from build123d import *

# Parameters (mm, degrees)
CROQUIS1_R              = 6
CROQUIS1_R_2            = 13
SALIENTE_EXTRUIR1_DEPTH = 9.525
CROQUIS2_R              = 13
CROQUIS2_R_2            = 7.5
SALIENTE_EXTRUIR2_DEPTH = 1.525


with BuildPart() as part:
    # Croquis1 → Saliente-Extruir1 (new body)
    with BuildSketch(Plane.XY):
        with BuildLine():
            Line((0, 19), (120, 19))
            ThreePointArc((120, 19), (139, 0), (120, -19))
            Line((120, -19), (0, -19))
            ThreePointArc((0, -19), (-19, 0), (0, 19))
        make_face()
        with Locations(Location((0, 0, 0), (0, 0, 180))):
            Circle(CROQUIS1_R, mode=Mode.SUBTRACT)
        with Locations(Location((120, 0, 0), (0, 0, 180))):
            Circle(CROQUIS1_R_2, mode=Mode.SUBTRACT)
    extrude(amount=SALIENTE_EXTRUIR1_DEPTH)

    # Croquis2 → Saliente-Extruir2 (add)
    with BuildSketch(Plane(origin=(0, 0, 0), x_dir=(-1, 0, 0), z_dir=(0, 0, -1))):
        with Locations((-120, 0)):
            Circle(CROQUIS2_R)
        with Locations((-120, 0)):
            Circle(CROQUIS2_R_2, mode=Mode.SUBTRACT)
    extrude(amount=-SALIENTE_EXTRUIR2_DEPTH)


solid = part.part
The listing builds one solid part. Answer for the finished solid, in the listing's coordinates (mm). A direction names the side the tool comes from. Round coordinates to 2 decimals unless told otherwise and drop trailing zeros. Order: outer loops, then holes, each group sorted by start corner. A loop starts at its lowest first (then second) coordinate and runs counter-clockwise, first axis right, second up. Notation, with made-up numbers: M 15.25,-21 L 44.25,-21 A29 ccw 44.25,4 Z; hole C -20.75,51 d10. An arc over 180 degrees is marked long. Answer in a Markdown table with one row per item. Add a question column.
1) Consider line 1 along Y through (x, z) = (120, 3.5); line 2 along Y through (x, z) = (0, 6.25); line 3 along X through (y, z) = (-5, 1.25). Determine where each line is inside the solid, lowest interval first. Write a range as from..to.
2) The part is cut by section B-B on z = 4.25. Determine the outline of the cut face in (x, y), plus the area to 3 significant figures.
3) Flat-ended cylindrical pins translate along their axes: pin 1 Ø4 at (y, z) = (14.5, 2.5) entering from +X; pin 2 Ø12 at (x, y) = (120, 0) entering from -Z; pin 3 Ø5 at (y, z) = (-3.5, 6.5) entering from +X; pin 4 Ø8 at (x, y) = (114, 6.5) entering from +Z (3 decimals). Find the tip coordinate at first contact, or state that the pin passes through.
4) The part is cut by section D-D on y = -16. Determine the outline of the cut face in (x, z) (3 decimals).
5) The part is cut by section C-C on x = -4. Determine the outline of the cut face in (y, z) (3 decimals), plus the area to 3 significant figures.
6) The part is cut by section A-A on y = 0. Determine the outline of the cut face in (x, z) (3 decimals), plus the area to 3 significant figures.
7) Which of the six approach directions +Z, -Z, +X, -X, +Y, -Y give full straight-line access (tool end or side, diameter ignored) to faces 1 (the face through (114, -6, 1.525)), 2 (the face through (-19, 0, 5))?
8) Determine the mould class of faces 3 (the face through (59, 19, 5)), 4 (the face through (61, 0, 0)), 5 (the face through (61, 0, 9.525)) for opening direction Z: pulls with the +Z half, pulls with the -Z half, needs draft (parallel to the pull), parting line crosses it, or undercut.
Findings below:
| question | item | result |
|---|---|---|
| 1 | line 1 | y = -19..-13, 13..19 |
| 1 | line 2 | y = -19..-6, 6..19 |
| 1 | line 3 | x = -18.33..-3.32, 3.32..114.41, 125.59..138.33 |
| 2 | outline | M 0,-19 L 120,-19 A19 ccw 120,19 L 0,19 A19 ccw Z; hole C 0,0 d12; hole C 120,0 d26 |
| 2 | area | 5,050 mm² |
| 3 | pin 1 | stops at x = 134.31 |
| 3 | pin 2 | passes through |
| 3 | pin 3 | stops at x = 138.97 |
| 3 | pin 4 | stops at z = 1.525 |
| 4 | outline | M -10.247,0 L 130.247,0 L 130.247,9.525 L -10.247,9.525 Z |
| 5 | outline | M -18.574,0 L -4.472,0 L -4.472,9.525 L -18.574,9.525 Z; M 4.472,0 L 18.574,0 L 18.574,9.525 L 4.472,9.525 Z |
| 5 | area | 269 mm² |
| 6 | outline | M -19,0 L -6,0 L -6,9.525 L -19,9.525 Z; M 6,0 L 112.5,0 L 112.5,1.525 L 107,1.525 L 107,9.525 L 6,9.525 Z; M 127.5,0 L 139,0 L 139,9.525 L 133,9.525 L 133,1.525 L 127.5,1.525 Z |
| 6 | area | 1,160 mm² |
| 7 | face 1 | +Z |
| 7 | face 2 | +Z, -Z, -X |
| 8 | face 3 | needs draft |
| 8 | face 4 | pulls with the -Z half |
| 8 | face 5 | pulls with the +Z half |
